```python
from build123d import *

# Parameters (mm, degrees)
SKETCH1_W           = 20
SKETCH1_H           = 30
BOSS_EXTRUDE1_DEPTH = 40
BOSS_EXTRUDE2_DEPTH = 5
SKETCH3_R           = 3.5
CUT_EXTRUDE1_DEPTH  = 41
SKETCH4_W           = 1.2
SKETCH4_H           = 40
CUT_EXTRUDE2_DEPTH  = 0.8


with BuildPart() as part:
    # Sketch1 → Boss-Extrude1 (new body)
    with BuildSketch(Plane(origin=(0, 0, 0), x_dir=(1, 0, 0), z_dir=(0, 1, 0))):
        with Locations((10, 15)):
            Rectangle(SKETCH1_W, SKETCH1_H)
    extrude(amount=BOSS_EXTRUDE1_DEPTH)

    # Sketch2 → Boss-Extrude2 (add)
    with BuildSketch(Plane(origin=(0, 40, 0), x_dir=(1, 0, 0), z_dir=(0, 1, 0))):
        Polygon((20, 0), (20, 3), (3, 3), (3, 27), (20, 27), (20, 30), (0, 30), (0, 0), align=None)
    extrude(amount=BOSS_EXTRUDE2_DEPTH)

    # Sketch3 → Cut-Extrude1 (cut, through all)
    with BuildSketch(Plane(origin=(0, 40, 0), x_dir=(1, 0, 0), z_dir=(0, 1, 0))):
        with Locations((14, 15)):
            Circle(SKETCH3_R)
        Polygon((12.582903769, 8.5), (10.562177826, 12), (6.520725942, 12), (4.5, 8.5), (6.520725942, 5), (10.562177826, 5), align=None)
        Polygon((12.582903769, 21.5), (10.562177826, 25), (6.520725942, 25), (4.5, 21.5), (6.520725942, 18), (10.562177826, 18), align=None)
    extrude(amount=-CUT_EXTRUDE1_DEPTH, mode=Mode.SUBTRACT)

    # Sketch4 → Cut-Extrude2 (cut)
    with BuildSketch(Plane(origin=(20, 0, 0), x_dir=(0, 0, -1), z_dir=(1, 0, 0))):
        with Locations((15, 20)):
            Rectangle(SKETCH4_W, SKETCH4_H)
    extrude(amount=-CUT_EXTRUDE2_DEPTH, mode=Mode.SUBTRACT)


solid = part.part
```
For this review, take the finished solid that the model builds, in its own axes (mm). A direction names the side the tool comes from. Give positions to 0.01 mm unless a question says otherwise; leave off trailing zeros. Order: outer loops, then holes, each group sorted by start corner. A loop starts at its lowest first (then second) coordinate and runs counter-clockwise, first axis right, second up.
1) Take a section at A-A (z = -15). Give the boundary of the cut face in (x, y).
2) Take a section at D-D (x = 5). Give the boundary of the cut face in (y, z).
3) The part is to be moulded in two halves that separate along Z. For faces 1 (the face through (10, 22, 0)), 2 (the face through (5.5, 20.28, -6.77)), 3 (the face through (20, 22, -7)), 4 (the face through (10, 22, -30)), say which applies: released by +Z, released by -Z, zero draft, split by the parting line, or undercut.
4) Take a section at C-C (y = 3.5). Give the boundary of the cut face in (x, z).
5) For faces 5 (the face through (19.2, 20, -15)), 6 (the face through (11, 42, -27)), 7 (the face through (0, 22, -15)), 8 (the face through (5.5, 20.28, -19.77)), list the 3-axis set-ups (+Z, -Z, +X, -X, +Y, -Y) from which the entire face can be reached by the end or side of a thin tool; tool diameter is ignored.
6) Wall thickness on line 1 (Z direction, x = 8.5, y = 13.5); line 2 (X direction, y = 2, z = -15); line 3 (Z direction, x = 13.75, y = 9): over which ranges is each line inside the solid? List them lowest first.
7) Insertion check: pin 1 (8.5 mm diameter, centred on x = 11.5, z = -20, fed in from +Y); pin 2 (0.6 mm diameter, centred on y = 21, z = -15, fed in from +X); pin 3 (2.5 mm diameter, centred on y = 43, z = -12.5, fed in from +X). Each pin has a flat end and moves straight along its axis. Give the tip position at first contact, or say it passes through.
8) Take a section at B-B (x = 14). Give the boundary of the cut face in (y, z).
Derived:
1. outline: (0, 0) - (10.5, 0) - (10.5, 40) - (3, 40) - (3, 45) - (0, 45) - close; (17.5, 0) - (19.2, 0) - (19.2, 40) - (17.5, 40) - close
2. outline: (0, -30) - (45, -30) - (45, -27) - (40, -27) - (40, -22.37) - (0, -22.37) - close; (0, -20.63) - (40, -20.63) - (40, -9.37) - (0, -9.37) - close; (0, -7.63) - (40, -7.63) - (40, -3) - (45, -3) - (45, 0) - (0, 0) - close
3. face 1: released by +Z
3. face 2: undercut
3. face 3: zero draft
3. face 4: released by -Z
4. outline: (0, -30) - (20, -30) - (20, -15.6) - (19.2, -15.6) - (19.2, -14.4) - (20, -14.4) - (20, 0) - (0, 0) - close; hole (4.5, -21.5) - (6.52, -25) - (10.56, -25) - (12.58, -21.5) - (10.56, -18) - (6.52, -18) - close; hole (4.5, -8.5) - (6.52, -12) - (10.56, -12) - (12.58, -8.5) - (10.56, -5) - (6.52, -5) - close; hole circle Ø7 at (14, -15)
5. face 5: +X, +Y, -Y
5. face 6: +X, +Y
5. face 7: +Z, -Z, -X, +Y, -Y
5. face 8: +Y, -Y
6. line 1: z = -30 to -25, -18 to -12, -5 to 0
6. line 2: x = 0 to 10.5, 17.5 to 19.2
6. line 3: z = -30 to -18.49, -11.51 to 0
7. pin 1: stops at y = 40
7. pin 2: stops at x = 19.2
7. pin 3: stops at x = 3
8. outline: (0, -30) - (45, -30) - (45, -27) - (40, -27) - (40, -18.5) - (0, -18.5) - close; (0, -11.5) - (40, -11.5) - (40, -3) - (45, -3) - (45, 0) - (0, 0) - close
